```python
from build123d import *

# Parameters (mm, degrees)
SKETCH1_R           = 3.96875
SKETCH1_R_2         = 15.08125
SKETCH1_R_3         = 2
BOSS_EXTRUDE1_DEPTH = 6.35


with BuildPart() as part:
    # Sketch1 → Boss-Extrude1 (new body)
    with BuildSketch(Plane(origin=(0, 0, 0), x_dir=(1, 0, 0), z_dir=(0, 1, 0))):
        with BuildLine():
            Line((25.4, -82.038158574), (25.4, -202.708825791))
            ThreePointArc((25.4, -202.708825791), (24.549261314, -205.883825791), (22.225, -208.208087105))
            Line((22.225, -208.208087105), (-19.685, -232.404836886))
            ThreePointArc((-19.685, -232.404836886), (-23.495, -232.404836886), (-25.4, -229.105280098))
            Line((-25.4, -229.105280098), (-25.4, -131.278691098))
            Line((-25.4, -131.278691098), (-6.917767735, 0.966806375))
            ThreePointArc((-6.917767735, 0.966806375), (-0.279220673, 6.97941694), (6.818426198, 1.51634072))
            Line((6.818426198, 1.51634072), (25.4, -82.038158574))
        make_face()
        with Locations(Location((0, 0, 0), (0, 0, 270))):
            Circle(SKETCH1_R, mode=Mode.SUBTRACT)
        with Locations(Location((0, -160.246508934, 0), (0, 0, 270))):
            Circle(SKETCH1_R_2, mode=Mode.SUBTRACT)
        with Locations(Location((-20.32, -225.425, 0), (0, 0, 270))):
            Circle(SKETCH1_R_3, mode=Mode.SUBTRACT)
        with Locations(Location((-20.32, -219.075, 0), (0, 0, 270))):
            Circle(SKETCH1_R_3, mode=Mode.SUBTRACT)
        with Locations(Location((-20.32, -212.725, 0), (0, 0, 270))):
            Circle(SKETCH1_R_3, mode=Mode.SUBTRACT)
        with Locations(Location((-20.32, -206.375, 0), (0, 0, 270))):
            Circle(SKETCH1_R_3, mode=Mode.SUBTRACT)
        with Locations(Location((0, -12.7, 0), (0, 0, 270))):
            Circle(SKETCH1_R_3, mode=Mode.SUBTRACT)
        with Locations(Location((19.05, -202.708825791, 0), (0, 0, 270))):
            Circle(SKETCH1_R_3, mode=Mode.SUBTRACT)
    extrude(amount=-BOSS_EXTRUDE1_DEPTH)


solid = part.part
```
For this review, take the finished solid that the model builds, in its own axes (mm). Round coordinates to 2 decimals unless told otherwise and drop trailing zeros. Loops run counter-clockwise (first coordinate to the right, second up) from the corner with the lowest first, then second, coordinate; pieces in that order, holes last.
(1) We need section A-A (y = -2). State how many separate pieces and enclosed holes the cut face has, plus the area to 3 significant figures.
Returned:
separate pieces: 1
enclosed holes: 8
area: 8,500 mm2
(2) Clearance check with flat-ended pins moving along their axes: P1, Ø3, axis at x = -7, y = -4, coming from the +Z side; P2, Ø1.5, axis at x = 9.5, y = -4, coming from the +Z side. State where each tip first meets the part, or that it passes through.
Returned:
P1: stops at z = 225.95
P2: stops at z = 215.99
(3) Wall thickness on line 1 along Z through (x, y) = (-3.5, -5.75); line 2 along X through (y, z) = (-3.5, 0); line 3 along X through (y, z) = (-6, 154.5): over which ranges is each line inside the solid? List them lowest first.
Returned:
line 1: z = -6.04 to -1.87, 1.87 to 145.58, 174.92 to 223.06
line 2: x = -7.05 to -3.97, 3.97 to 7.16
line 3: x = -25.4 to -13.94, 13.94 to 25.4
(4) Mouldability with a two-part tool opening along Z and no side actions: class faces 1 (the cylindrical face through (-0.766, -3.131, 14.547)), 2 (the cylindrical face through (-0.415, -3.131, -6.973)), 3 (the flat face through (0, 0, 111)), 4 (the cylindrical face through (-23.45, -3.13, 232.43)) as released by +Z, released by -Z, zero draft, split by the parting line, or undercut.
Returned:
face 1: undercut
face 2: released by -Z
face 3: zero draft
face 4: released by +Z
(5) We need section C-C (x = 0). Give the boundary of the cut face in (y, z) (3 decimals), plus the area to 3 significant figures.
Returned:
outline: (-6.35, -6.985) - (0, -6.985) - (0, -3.969) - (-6.35, -3.969) - close; (-6.35, 3.969) - (0, 3.969) - (0, 10.7) - (-6.35, 10.7) - close; (-6.35, 14.7) - (0, 14.7) - (0, 145.165) - (-6.35, 145.165) - close; (-6.35, 175.328) - (0, 175.328) - (0, 221.04) - (-6.35, 221.04) - close
area: 1,180 mm2
(6) We need section D-D (z = 34.5). Give the boundary of the cut face in (x, y), plus the area to 3 significant figures.
Returned:
outline: (-11.87, -6.35) - (14.83, -6.35) - (14.83, 0) - (-11.87, 0) - close
area: 170 mm2
(7) We need section B-B (x = 13). Give the boundary of the cut face in (y, z).
Returned:
outline: (-6.35, 26.28) - (0, 26.28) - (0, 152.6) - (-6.35, 152.6) - close; (-6.35, 167.89) - (0, 167.89) - (0, 213.53) - (-6.35, 213.53) - close
